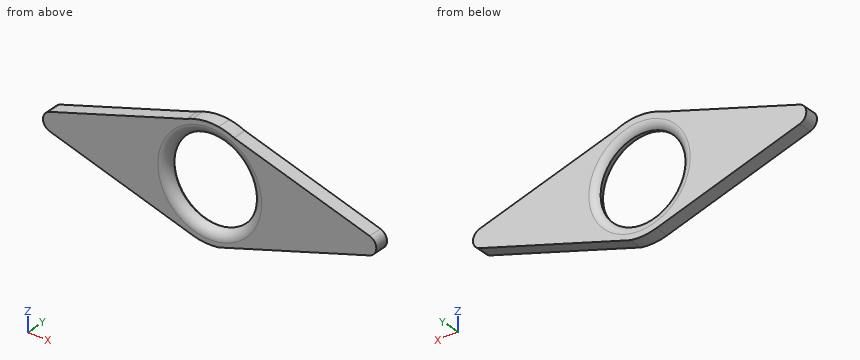
```python
from build123d import *

# Parameters (mm, degrees)
F0_R     = 11.43
F1_DEPTH = 3.81
F2_R     = 2.54


# Not quite as in the source:
# - a fillet or chamfer that OpenCascade refuses, or shapes differently, is made with other operations: its cross-section is extruded or revolved along the edge and cut away or added


with BuildPart() as f1:
    # F0 (on Front) → F1 (new body)
    with BuildSketch(Plane.XZ):
        with BuildLine():
            Line((6.5569237481, 13.7573380769), (2.4006070358, 15.0497403918))
            ThreePointArc((2.4006070358, 15.0497403918), (-1.1592691439, 15.195844664), (-4.6557853401, 14.5114183617))
            ThreePointArc((-4.6557853401, 14.5114183617), (-5.4590945375, 14.2286994076), (-6.2453574463, 13.9015506462))
            Line((-6.2453574463, 13.9015506462), (-50.8, 0))
            Line((-50.8, 0), (-4.5719998884, -14.5380334647))
            ThreePointArc((-4.5719998884, -14.5380334647), (-1.1154361142, -15.1991250497), (2.4006070358, -15.0497403918))
            Line((2.4006070358, -15.0497403918), (50.8, 0))
            Line((50.8, 0), (6.5569237481, 13.7573380769))
        make_face()
        Circle(F0_R, mode=Mode.SUBTRACT)
        with BuildLine():
            ThreePointArc((6.5569237481, 13.7573380769), (4.5251425803, 14.552686509), (2.4006070358, 15.0497403918))
            Line((2.4006070358, 15.0497403918), (6.5569237481, 13.7573380769))
        make_face()
    extrude(amount=F1_DEPTH)

    # F2
    f2_edges = [f1.edges().sort_by_distance(p)[0] for p in [
        (50.8, -1.905, 0),
        (-50.8, -1.905, 0),
        (-11.43, -3.81, 0),
    ]]
    fillet(f2_edges, radius=F2_R)

    # F3: fillet of radius 2.54 on 1 edges, made by hand

    # F3_s1 → F3_t2 (revolve, cut)
    with BuildSketch(Plane.XY):
        with BuildLine():
            ThreePointArc((13.6297045256, 0), (12.3597045256, -0.3402954744), (11.43, -1.27))
            Line((11.43, -1.27), (11.43, 0))
            Line((11.43, 0), (13.6297045256, 0))
        make_face()
    revolve(axis=Axis((0, 0, 0), (0, -1, 0)), mode=Mode.SUBTRACT)


solid = f1.part
```
Could you check a few things on this model? Use its own coordinates, in mm. Round coordinates to 2 decimals unless told otherwise and drop trailing zeros. Write each loop counter-clockwise with the first axis right and the second up, starting at its lowest first coordinate (ties: lowest second). Pieces come first, ordered by that corner, then holes. Notation, with made-up numbers: M 31.5,-29.5 L 83.5,-29.5 A26 cw 83.5,1.5 Z; hole C 1.25,18 d11. An arc over 180 degrees is marked long. Write each question's results on one line, items separated by ' | '. Start each with the question number.
1. Imagine slicing it at B-B on x = 21.5. List the corners of the cut face in (y, z) for me, and give its area (3 significant figures).
2. I need wall thicknesses on L1, parallel to Z at x = -1, y = -2.8; L2, parallel to Y at x = -2.5, z = -13.5; L3, parallel to Z at x = 3, y = -3.2. Which ranges of each line are inside material? Lowest first, please. Write a range as from..to.
3. Imagine slicing it at A-A on y = -2.25. List the corners of the cut face in (x, z) for me, and give its area (3 significant figures).
4. I'm going to push flat-ended pins straight in: pin 1 Ø8 at (x, z) = (-8, 4) entering from +Y; pin 2 Ø2 at (x, y) = (20, -1.5) entering from -Z. Where does each tip first touch, or does it pass through?
Result sheet:
1) outline: M -3.81,-9.11 L 0,-9.11 L 0,9.11 L -3.81,9.11 Z | area: 69.4 mm^2
2) L1: z = -15.21..-11.9, 11.9..15.21 | L2: y = -3.8..0 | L3: z = -14.86..-11.95, 11.95..14.94
3) outline: M -43.06,-2.43 L -4.57,-14.54 A15.24 ccw 2.4,-15.05 L 43,-2.43 A2.54 ccw 43,2.43 L 6.56,13.76 A15.24 ccw -6.25,13.9 L -43.06,2.42 A2.54 ccw Z; hole C 0,0 d23.25 | area: 1,160 mm^2
4) pin 1: stops at y = -0.09 | pin 2: stops at z = -9.89
